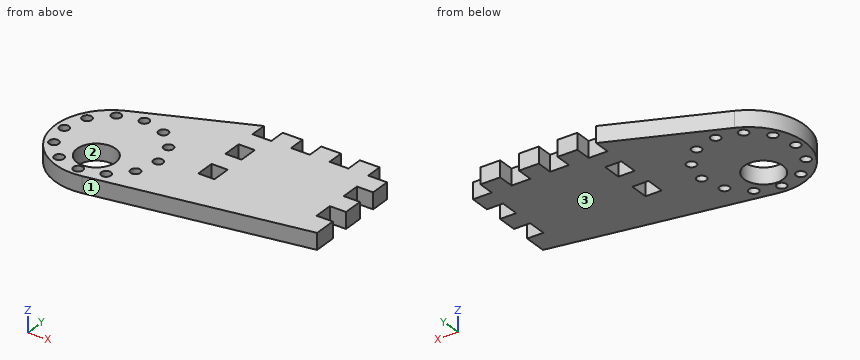
from build123d import *

# Parameters (mm, degrees)
BOSS_EXTRUDE1_DEPTH          = 5.334
SKETCH1_3_R                  = 6.35
SKETCH1_3_R_2                = 6
CUT_EXTRUDE2_DEPTH           = 80.087198141
F_1_8_0_125_DIAMETER_HOLE1_D = 3.175
SKETCH4_W                    = 6.1976
SKETCH4_H                    = 5.334
CUT_EXTRUDE3_DEPTH           = 80.087198141
LPATTERN1_COUNT              = 4
LPATTERN1_PITCH              = 12.7
SKETCH5_W                    = 5.334
SKETCH5_H                    = 6.1976
CUT_EXTRUDE4_DEPTH           = 80.087198141
LPATTERN2_COUNT              = 2
LPATTERN2_PITCH              = 12.7


with BuildPart() as part:
    # Sketch1 → Boss-Extrude1 (new body)
    with BuildSketch(Plane.XY):
        with BuildLine():
            Line((72.2376, 31.75), (27.94, 31.75))
            Line((27.94, 31.75), (-7.148981901, 16.95441116))
            ThreePointArc((-7.148981901, 16.95441116), (-17.663197211, -5.154751622), (3.092321188, -18.138289602))
            Line((3.092321188, -18.138289602), (72.2376, -6.35))
            Line((72.2376, -6.35), (72.2376, 31.75))
        make_face()
    extrude(amount=BOSS_EXTRUDE1_DEPTH)

    # Sketch1_3 → Cut-Extrude2 (cut, through all)
    with BuildSketch(Plane.XY):
        with Locations((0, -7)):
            Circle(SKETCH1_3_R)
        with Locations((0, -7)):
            Circle(SKETCH1_3_R_2)
    extrude(amount=CUT_EXTRUDE2_DEPTH, mode=Mode.SUBTRACT)

    # 1_8 _0.125_ Diameter Hole1 (through all)
    with Locations(Plane.XY.offset(5.334)):
        with Locations((0, 15.5), (7.75, 13.423393759), (13.423393759, 7.75), (15.5, 0), (13.423393759, -7.75), (7.75, -13.423393759), (0, -15.5), (-7.75, -13.423393759), (-13.423393759, -7.75), (-15.5, 0), (-13.423393759, 7.75), (-7.75, 13.423393759)):
            Hole(F_1_8_0_125_DIAMETER_HOLE1_D / 2)

    # Sketch4 → Cut-Extrude3 (cut, through all)
    with BuildSketch(Plane.XY.offset(5.334)):
        with Locations((31.0388, 29.083)):
            Rectangle(SKETCH4_W, SKETCH4_H)
    cut_extrude3 = extrude(amount=-CUT_EXTRUDE3_DEPTH, mode=Mode.SUBTRACT)

    # LPattern1: Cut-Extrude3 ×4
    with Locations(*[(i * LPATTERN1_PITCH, 0, 0) for i in range(1, LPATTERN1_COUNT)]):
        add(cut_extrude3, mode=Mode.SUBTRACT)

    # Sketch5 → Cut-Extrude4 (cut, through all)
    with BuildSketch(Plane.XY.offset(5.334)):
        with Locations((69.5706, 16.8148)):
            Rectangle(SKETCH5_W, SKETCH5_H)
        with Locations((30.607, 16.8148)):
            Rectangle(SKETCH5_W, SKETCH5_H)
    cut_extrude4 = extrude(amount=-CUT_EXTRUDE4_DEPTH, mode=Mode.SUBTRACT)

    # LPattern2: Cut-Extrude4 ×2
    with Locations(*[(0, -i * LPATTERN2_PITCH, 0) for i in range(1, LPATTERN2_COUNT)]):
        add(cut_extrude4, mode=Mode.SUBTRACT)


solid = part.part
Work out the finished part from the listing and answer in its coordinate system (mm). Face numbers are marked on the shaded views. Give positions to 0.01 mm unless a question says otherwise; leave off trailing zeros. Write each loop counter-clockwise with the first axis right and the second up, starting at its lowest first coordinate (ties: lowest second). Pieces come first, ordered by that corner, then holes. Notation, with made-up numbers: M 50,77.25 L 64,77.25 A31 cw 64,113.25 Z; hole C 3.25,61.5 d6. An arc over 180 degrees is marked long. Answer as CSV lines item,"result".
Q1. A cutting plane is placed at B-B on y = 5. Write down the section's boundary in (x, z), plus the area to 3 significant figures.
A:
outline,"M -17.71,0 L 27.94,0 L 27.94,5.33 L -17.71,5.33 Z; M 33.27,0 L 66.9,0 L 66.9,5.33 L 33.27,5.33 Z"
area,"423 mm²"
Q2. Find the intervals of material crossed by probe 1 along Y at (x, z) = (29, 1); probe 2 along X at (y, z) = (-0.5, 3.75); probe 3 along Y at (x, z) = (0, 3.8), in increasing order. Write a range as [from, to].
A:
probe 1,"y = [-13.72, 1.02], [7.21, 13.72], [19.91, 26.42]"
probe 2,"x = [-18.39, -17.01], [-13.99, 13.99], [17.01, 72.24]"
probe 3,"y = [-18.4, -17.09], [-13.91, -13.35], [-0.65, 13.91], [17.09, 19.97]"
Q3. A cutting plane is placed at A-A on x = 7.75. Write down the section's boundary in (y, z), plus the area to 3 significant figures.
A:
outline,"M -17.34,0 L -15.01,0 L -15.01,5.33 L -17.34,5.33 Z; M -11.84,0 L 11.84,0 L 11.84,5.33 L -11.84,5.33 Z; M 15.01,0 L 23.24,0 L 23.24,5.33 L 15.01,5.33 Z"
area,"183 mm²"
Q4. The mould has two halves that part along X. Classify the marked faces 1, 2 and 3: +X half, -X half, draft (parallel to the pull), parting line (faces both ways), or undercut.
A:
face 1,"+X half"
face 2,"undercut"
face 3,"draft"
Q5. A cutting plane is placed at D-D on z = 2.3. Count the separate pieces of the cut face and the enclosed holes in it, plus the area to 3 significant figures.
A:
separate pieces,"1"
enclosed holes,"15"
area,"3,080 mm²"
Q6. Given P1, Ø3, axis at x = 15.5, y = 0, coming from the -Z side; P2, Ø2.5, axis at x = 30, z = 2.5, coming from the -Y side; P3, Ø3, axis at y = -8, z = 1.5, coming from the -X side; P4, Ø2.5, axis at y = 29, z = 3, coming from the +X side, each flat-ended and moving along its own axis, determine where each tip first touches the part or whether it passes through.
A:
P1,"passes through"
P2,"stops at y = -13.76"
P3,"stops at x = -17.21"
P4,"stops at x = 66.04"
Q7. A cutting plane is placed at C-C on x = -3.5. Write down the section's boundary in (y, z).
A:
outline,"M -18.06,0 L -12.3,0 L -12.3,5.33 L -18.06,5.33 Z; M -1.7,0 L 18.49,0 L 18.49,5.33 L -1.7,5.33 Z"
